Part model, mm, in its own coordinate system. A direction names the side the tool comes from. Coordinates: 2 decimals unless noted, no trailing zeros. Loops run counter-clockwise (first coordinate to the right, second up) from the corner with the lowest first, then second, coordinate; pieces in that order, holes last. Notation, with made-up numbers: M 24,35.25 L 53,35.25 A21 ccw 53,62.25 Z; hole C 39.25,-2 d6. An arc over 180 degrees is marked long. Use CSV: the item, a comma, the result in double quotes. Start each with the question number.
Solid Edge part; units mm, degrees
sketch "Sketch1" plane through (0, 50, 11.75) normal (0, -1, 0) x (1, 0, 0)
  line L0 (-27.5, -33.25) -> (27.5, -33.25)
  line L1 (27.5, 9.75) -> (27.5, -33.25)
  line L2 (27.5, 9.75) -> (-27.5, 9.75)
  line L3 (-27.5, 9.75) -> (-27.5, -33.25)
  dimension "D1" = 27.5
  dimension "D2" = 27.5
extrude "ExtrudedProtrusion_2" add sketch "Sketch1" along normal blind 12
sketch "Sketch2" plane through (0, 0, 0) normal (1, 0, 0) x (0, 1, 0)
  arc A0 (50, -9.5) -> (50, 9.5) centre (50, 0) cw
  line L0 (50, 9.5) -> (50, -9.5)
  dimension "D1" = 50
extrude "Cutout1" cut sketch "Sketch2" along normal through all and the other way through all
sketch "Sketch3" plane through (-27.5, 44, 0) normal (-1, 0, 0) x (0, 0, -1)
  line L0 (27.9876, -6) -> (21.5, -6)
  line L1 (21.5, -6) -> (21.5, 1.5)
  arc A0 (-21.5, 1.5) -> (21.5, 1.5) centre (0, -48.0353) cw
  line L2 (-21.5, -6) -> (-21.5, 1.5)
  line L3 (-21.5, -6) -> (-27.4197, -6)
  line L4 (-27.4197, -6) -> (-27.4197, 18.1819)
  line L5 (-27.4197, 18.1819) -> (27.9876, 18.1819)
  line L6 (27.9876, 18.1819) -> (27.9876, -6)
extrude "Cutout2" cut sketch "Sketch3" against normal up to next
sketch "Sketch4" plane through (0, 38, 0) normal (0, -1, 0) x (1, 0, 0)
  circle A0 centre (-18.5, -14) radius 3
  circle A1 centre (18.5, -14) radius 3
  circle A2 centre (18.5, 14) radius 3
  circle A3 centre (-18.5, 14) radius 3
  dimension "D1" = 18.5
  dimension "D2" = 18.5
extrude "Cutout3" cut sketch "Sketch4" against normal through all
sketch "Sketch5" plane through (0, 38, 0) normal (0, -1, 0) x (1, 0, 0)
  circle A0 centre (-18.5, 14) radius 7
  circle A1 centre (18.5, 14) radius 7
  circle A2 centre (-18.5, -14) radius 7
  circle A3 centre (18.5, -14) radius 7
extrude "Cutout4" cut sketch "Sketch5" against normal blind 4.5
sketch "Sketch6" plane through (0, 38, 0) normal (0, -1, 0) x (1, 0, 0)
  arc A0 (11, -22.0467) -> (7.5, -14) centre (18.5, -14) cw
  line L0 (-7.5, -14) -> (7.5, -14)
  arc A1 (-11, -22.0467) -> (-7.5, -14) centre (-18.5, -14) ccw
  line L1 (-11, -22.0467) -> (11, -22.0467)
  line L2 (-11, 22.0467) -> (11, 22.0467)
  arc A2 (7.5, 14) -> (11, 22.0467) centre (18.5, 14) cw
  line L3 (-7.5, 14) -> (7.5, 14)
  arc A3 (-7.5, 14) -> (-11, 22.0467) centre (-18.5, 14) ccw
  dimension "D1" = 7.5
  dimension "D2" = 11
extrude "ExtrudedCutout_9" cut sketch "Sketch6" against normal blind 10
properties material "Aluminum, 1060"
1. Slice it at C-C, the plane z = 12.5. List the corners of the cut face in (x, y), and give its area (3 significant figures).
2. Slice it at B-B, the plane x = -20.5. List the corners of the cut face in (y, z).
3. Two-plate mould, pull along Z, no slides. Class faces 1 (the face through (0, 48, 18)), 2 (the face through (15, 42.5, -14)), 3 (the face through (-8.244, 44.786, 17.976)), 4 (the face through (15, 42.5, 14)): pulls with the +Z half, pulls with the -Z half, needs draft (parallel to the pull), parting line crosses it, or undercut.
4. Pin check, flat tips, straight feed: pin 1 (11 mm diameter, centred on x = 18.5, z = -14, fed in from -Y); pin 2 (6.5 mm diameter, centred on x = 3, y = 42.5, fed in from +Z); pin 3 (15.5 mm diameter, centred on x = 20.5, z = -14, fed in from -Y). Stop position of each tip, or through.
5. Slice it at D-D, the plane x = 6.5. List the corners of the cut face in (y, z), and give its area (3 significant figures).
6. Wall check: probe 1 along Z at (x, y) = (21, 48); probe 2 along X at (y, z) = (41.5, -11.5); probe 3 along Z at (x, y) = (-22, 49.5). Give the ranges that are in metal, low to high.
7. Slice it at A-A, the plane y = 45. List the corners of the cut face in (x, z).
8. Tool access for faces 5 (the face through (8.244, 44.786, -17.976)), 6 (the face through (17.59, 40.91, -7.06)), 7 (the face through (27.5, 40, 0)), 8 (the face through (0, 44, 14)): list every direction of +Z, -Z, +X, -X, +Y, -Y with a clear straight run to the whole face (end or side of a thin tool).
Found:
1,outline,"M -27.5,39.5 L -25.34,39.5 L -25.34,42.5 L -21.1,42.5 L -21.1,50 L -27.5,50 Z; M -15.9,42.5 L -11.66,42.5 L -11.66,39.5 L 11.66,39.5 L 11.66,42.5 L 15.9,42.5 L 15.9,50 L -15.9,50 Z; M 21.1,42.5 L 25.34,42.5 L 25.34,39.5 L 27.5,39.5 L 27.5,50 L 21.1,50 Z"
1,area,"417 mm^2"
2,outline,"M 38.53,-7.29 L 42.5,-7.29 L 42.5,-11.76 L 50,-11.76 L 50,-9.5 A9.5 cw 50,9.5 L 50,11.76 L 42.5,11.76 L 42.5,7.29 L 38.53,7.29 A54 ccw Z; M 42.16,-20.71 A54 ccw 42.5,-21.5 L 50,-21.5 L 50,-16.24 L 42.5,-16.24 L 42.5,-20.71 Z; M 42.16,20.71 L 42.5,20.71 L 42.5,16.24 L 50,16.24 L 50,21.5 L 42.5,21.5 A54 ccw Z"
3,face 1,"needs draft"
3,face 2,"undercut"
3,face 3,"pulls with the +Z half"
3,face 4,"undercut"
4,pin 1,"y = 42.5"
4,pin 2,"z = 14"
4,pin 3,"y = 38.4"
5,outline,"M 39.88,-14 L 48,-14 L 48,-21.5 L 50,-21.5 L 50,-9.5 A9.5 cw 50,9.5 L 50,21.5 L 48,21.5 L 48,14 L 39.88,14 A54 ccw Z"
5,area,"206 mm^2"
6,probe 1,"-21.5 to -15.66, -12.34 to -9.29, 9.29 to 12.34, 15.66 to 21.5"
6,probe 2,"-27.5 to -25.04, -11.96 to 11.96, 25.04 to 27.5"
6,probe 3,"-21.5 to -9.49, 9.49 to 21.5"
7,outline,"M -27.5,-21.5 L -10.45,-21.5 A11 ccw -7.5,-14 L 7.5,-14 A11 ccw 10.45,-21.5 L 27.5,-21.5 L 27.5,-8.08 L -27.5,-8.08 Z; M -27.5,8.08 L 27.5,8.08 L 27.5,21.5 L 10.45,21.5 A11 ccw 7.5,14 L -7.5,14 A11 ccw -10.45,21.5 L -27.5,21.5 Z; hole C -18.5,-14 d6; hole C -18.5,14 d6; hole C 18.5,-14 d6; hole C 18.5,14 d6"
8,face 5,"-Z, -Y"
8,face 6,"-Y"
8,face 7,"+Z, -Z, +X, +Y, -Y"
8,face 8,"+Z, -Y"
